Here's how the part is built. I have some questions about the finished solid (model axes, mm). Face numbers are marked on the shaded views. A direction names the side the tool comes from. Round coordinates to 2 decimals unless told otherwise and drop trailing zeros. Loops run counter-clockwise (first coordinate to the right, second up) from the corner with the lowest first, then second, coordinate; pieces in that order, holes last. Notation, with made-up numbers: M 71,2 L 75,2 A21 ccw 75,24 Z; hole C 47,27 d3. An arc over 180 degrees is marked long. Answer as CSV lines item,"result".
```python
from build123d import *

# Parameters (mm, degrees)
SKETCH1_W           = 44.8
SKETCH1_H           = 4.8
BOSS_EXTRUDE1_DEPTH = 16.8
FILLET1_R           = 5
CUT_EXTRUDE1_DEPTH  = 32.95768929
SKETCH3_W           = 1.2
SKETCH3_H           = 13
BOSS_EXTRUDE2_DEPTH = 3
SKETCH4_W           = 16.8
SKETCH4_H           = 1.2
BOSS_EXTRUDE3_DEPTH = 2
SKETCH5_R           = 1
BOSS_EXTRUDE4_DEPTH = 2
FILLET2_R           = 2


with BuildPart() as part:
    # Sketch1 → Boss-Extrude1 (new body)
    with BuildSketch(Plane.XY):
        with Locations((4.109677419, 3.624193548)):
            Rectangle(SKETCH1_W, SKETCH1_H)
    extrude(amount=BOSS_EXTRUDE1_DEPTH)

    # Fillet1
    # the kernel refuses this fillet: 5 mm, written as the material it takes off along each edge
    with BuildSketch(Plane(origin=(26.509677419, 6.024193548, -12.489995997), x_dir=(-1, 0, 0), z_dir=(0, 0, 1))) as fillet1_piece_1:
        with BuildLine():
            CenterArc((4.995998399, 5), FILLET1_R, 182.292442776, 87.707557224)
            Line((0, 4.8), (-0.099919968, 4.796))
            ThreePointArc((-0.099919968, 4.796), (-0.1, 2.4), (-0.1, 0))
            Line((-0.1, 0), (0, -0.1))
            Line((0, -0.1), (4.995998399, -0.1))
            Line((4.995998399, -0.1), (4.995998399, 0))
        make_face()
    extrude(amount=41.779991994, mode=Mode.SUBTRACT)

    # Sketch2 → Cut-Extrude1 (cut, through all)
    with BuildSketch(Plane(origin=(0, 0, 0), x_dir=(-1, 0, 0), z_dir=(0, 0, -1))):
        with BuildLine():
            Line((-24.1059753, 1.224193548), (18.290322581, 1.224193548))
            Line((18.290322581, 1.224193548), (18.290322581, 3.624193548))
            Line((18.290322581, 3.624193548), (-21.513679021, 3.624193548))
            ThreePointArc((-21.513679021, 3.624193548), (-23.280031194, 2.932071951), (-24.1059753, 1.224193548))
        make_face()
    extrude(amount=-CUT_EXTRUDE1_DEPTH, mode=Mode.SUBTRACT)

    # Sketch3 → Boss-Extrude2 (add)
    with BuildSketch(Plane.XZ.offset(-1.224193548)):
        with Locations((24.7059753, 6.5)):
            Rectangle(SKETCH3_W, SKETCH3_H)
    extrude(amount=BOSS_EXTRUDE2_DEPTH)

    # Sketch4 → Boss-Extrude3 (add)
    with BuildSketch(Plane.ZY.offset(18.290322581)):
        with Locations((8.4, 4.224193548)):
            Rectangle(SKETCH4_W, SKETCH4_H)
    extrude(amount=BOSS_EXTRUDE3_DEPTH)

    # Sketch5 → Boss-Extrude4 (add)
    with BuildSketch(Plane(origin=(0, 0, 0), x_dir=(-1, 0, 0), z_dir=(0, 0, -1))):
        with BuildLine():
            Line((-18.1059753, -0.775806452), (-18.1059753, 3.624193548))
            Line((-18.1059753, 3.624193548), (-21.513679021, 3.624193548))
            ThreePointArc((-21.513679021, 3.624193548), (-23.280031194, 2.932071951), (-24.1059753, 1.224193548))
            Line((-24.1059753, 1.224193548), (-24.1059753, -0.775806452))
            Line((-24.1059753, -0.775806452), (-18.1059753, -0.775806452))
        make_face()
        with Locations((-21.513679021, 1.024193548)):
            Circle(SKETCH5_R, mode=Mode.SUBTRACT)
    extrude(amount=-BOSS_EXTRUDE4_DEPTH)

    # Fillet2
    fillet2_edges = [part.edges().sort_by_distance(p)[0] for p in [
        (18.1059753, -0.775806452, 1),
    ]]
    fillet(fillet2_edges, radius=FILLET2_R)


solid = part.part
```
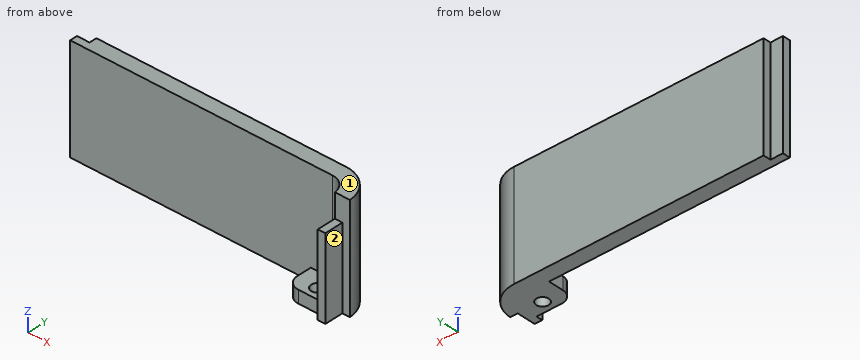
1. I want a section at B-B, the plane z = 1.25. Please give me the cut outline in (x, y).
Evaluation:
outline,"M -20.29,3.62 L 18.11,3.62 L 18.11,1.22 A2 ccw 20.11,-0.78 L 24.11,-0.78 L 24.11,-1.78 L 25.31,-1.78 L 25.31,1.22 L 26.51,1.22 A5 ccw 21.51,6.02 L -18.29,6.02 L -18.29,4.82 L -20.29,4.82 Z; hole C 21.51,1.02 d2"
2. For P1, Ø1.6, axis at x = -19, z = 9, coming from the +Y side; P2, Ø0.6, axis at y = 5.5, z = 7.5, coming from the -X side; P3, Ø2, axis at y = 4.5, z = 9.5, coming from the +X side; P4, Ø1, axis at y = 2.5, z = 5, coming from the +X side, each with a flat end and sliding along its axis, tell me the tip position at first contact or that it passes through.
Evaluation:
P1,"stops at y = 6.02"
P2,"stops at x = -18.29"
P3,"stops at x = 25.86"
P4,"stops at x = 26.42"
3. I want a section at A-A, the plane z = 7. Please give me the cut outline in (x, y), and give its area (3 significant figures).
Evaluation:
outline,"M -20.29,3.62 L 21.51,3.62 A2.6 cw 24.11,1.22 L 24.11,-1.78 L 25.31,-1.78 L 25.31,1.22 L 26.51,1.22 A5 ccw 21.51,6.02 L -18.29,6.02 L -18.29,4.82 L -20.29,4.82 Z"
area,"115 mm²"
4. Which directions (+Z, -Z, +X, -X, +Y, -Y) give clear straight access to the entire face, cutting with the end or side of a thin tool? Please do the marked faces 1 and 2.
Evaluation:
face 1,"+Z, +X, -X, +Y, -Y"
face 2,"+Z, -Z, +X, -Y"
5. If I drill on line 1 (X direction, y = 0, z = 6.5); line 2 (Y direction, x = -17, z = 11.5); line 3 (X direction, y = 0.5, z = 1.5), over which ranges is the centre line in solid material (lowest first)? Write a range as [from, to].
Evaluation:
line 1,"x = [24.11, 25.31]"
line 2,"y = [3.62, 6.02]"
line 3,"x = [18.24, 20.66], [22.37, 25.31]"
6. I want a section at D-D, the plane x = -11.5. Please give me the cut outline in (y, z), and give its area (3 significant figures).
Evaluation:
outline,"M 3.62,0 L 6.02,0 L 6.02,16.8 L 3.62,16.8 Z"
area,"40.3 mm²"
7. I want a section at C-C, the plane y = 3. Please give me the cut outline in (x, z).
Evaluation:
outline,"M 18.11,0 L 26.11,0 L 26.11,16.8 L 23.2,16.8 L 23.2,2 L 18.11,2 Z"
